Verification items for the finished model (mm, model axes). Face numbers are marked on the shaded views. Coordinates: 2 decimals unless noted, no trailing zeros. Order: outer loops, then holes, each group sorted by start corner. A loop starts at its lowest first (then second) coordinate and runs counter-clockwise, first axis right, second up.
Q1. Cross-section at B-B, the plane z = 10.5. Count the separate pieces of the cut face and the enclosed holes in it, and give its area (3 significant figures).
Q2. Cross-section at A-A, the plane x = 0. Record the boundary of the cut face in (y, z).
Q3. Thickness scan on line 1 (Y direction, x = 14, z = 10.25); line 2 (Y direction, x = 10.5, z = 9.75); line 3 (X direction, y = -21.5, z = 10.5). Record the ranges inside material, lowest first.
Q4. Draft check along Z on the marked faces 1, 2 and 3. Enter one of: pulls with the +Z half, pulls with the -Z half, needs draft (parallel to the pull), parting line crosses it, or undercut.
Q5. Depth check by flat-ended pin: P1, Ø4, axis at x = 4, z = 12, coming from the -Y side; P2, Ø2, axis at x = -5.5, z = 18, coming from the +Y side; P3, Ø15.5, axis at x = 0, y = 0, coming from the -Z side; P4, Ø5, axis at y = -14, z = 12.5, coming from the +X side. Enter the tip coordinate at first touch or a pass-through.
Q6. Cross-section at D-D, the plane z = 3.75. Record the boundary of the cut face in (x, y), and give its area (3 significant figures).
from build123d import *

# Parameters (mm, degrees)
SKETCH1_R           = 29.75
SKETCH1_R_2         = 12.928028004
BOSS_EXTRUDE1_DEPTH = 21
SKETCH3_R           = 3.81
CUT_EXTRUDE1_DEPTH  = 31
CIRPATTERN1_COUNT   = 10


with BuildPart() as part:
    # Sketch1 → Boss-Extrude1 (new body)
    with BuildSketch(Plane.XY):
        with Locations(Location((0, 0, 0), (0, 0, 180))):
            Circle(SKETCH1_R)
        with Locations(Location((0, 0, 0), (0, 0, 180))):
            Circle(SKETCH1_R_2, mode=Mode.SUBTRACT)
    extrude(amount=BOSS_EXTRUDE1_DEPTH)

    # Sketch3 → Cut-Extrude1 (cut)
    with BuildSketch(Plane(origin=(0, 0, 0), x_dir=(1, 0, 0), z_dir=(0, 1, 0))):
        with Locations(Location((0, -10.5, 0), (0, 0, 270))):
            Circle(SKETCH3_R)
    cut_extrude1 = extrude(amount=-CUT_EXTRUDE1_DEPTH, mode=Mode.SUBTRACT)

    # CirPattern1: Cut-Extrude1 ×10 about axis
    cirpattern1_axis = Axis((0, 0, 21), (0, 0, -1))
    for i in range(1, CIRPATTERN1_COUNT):
        add(cut_extrude1.rotate(cirpattern1_axis, i * 360 / CIRPATTERN1_COUNT), mode=Mode.SUBTRACT)


solid = part.part
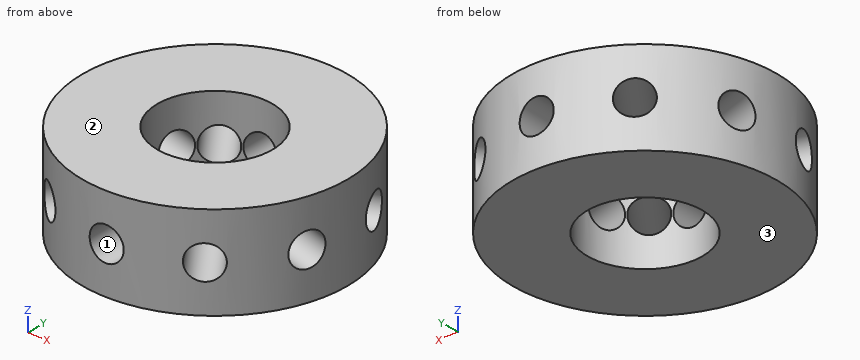
Check values:
1. separate pieces: 10
1. enclosed holes: 0
1. area: 965 mm2
2. outline: (-29.75, 0) - (-12.93, 0) - (-12.93, 6.69) - (-29.75, 6.69) - close; (-29.75, 14.31) - (-12.93, 14.31) - (-12.93, 21) - (-29.75, 21) - close; (12.93, 0) - (29.75, 0) - (29.75, 6.69) - (12.93, 6.69) - close; (12.93, 14.31) - (29.75, 14.31) - (29.75, 21) - (12.93, 21) - close
3. line 1: y = -26.25 to -25.74, -12.8 to -8.55, -0.55 to 0.55, 8.55 to 12.8, 25.74 to 26.25
3. line 2: y = -27.84 to -20.81, -8.1 to -7.54, 7.54 to 8.1, 20.81 to 27.84
3. line 3: x = -20.56 to -20.33, -10.91 to -3.81, 3.81 to 10.91, 20.33 to 20.56
4. face 1: undercut
4. face 2: pulls with the +Z half
4. face 3: pulls with the -Z half
5. P1: stops at y = -29.64
5. P2: stops at y = 29.41
5. P3: passes through
5. P4: stops at x = 27.38
6. outline: circle Ø59.5 at (0, 0); hole circle Ø25.86 at (0, 0)
6. area: 2,260 mm2
